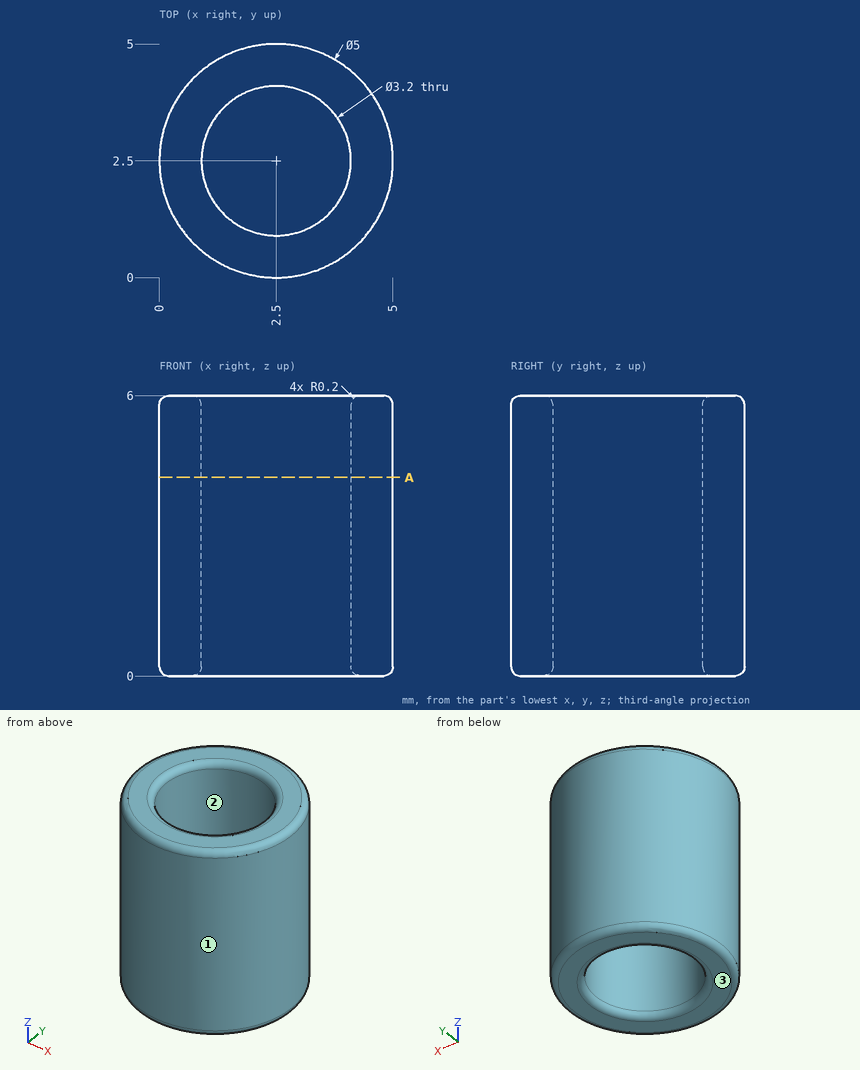
Study the drawing (mm; zero at the part's minimum x, y, z) and answer. Coordinates: 2 decimals unless noted, no trailing zeros. Write each loop counter-clockwise with the first axis right and the second up, starting at its lowest first coordinate (ties: lowest second). Pieces come first, ordered by that corner, then holes.
Q1. Given P1, Ø3, axis at x = 2.5, y = 2.5, coming from the +Z side; P2, Ø1.5, axis at x = 3.5, z = 4, coming from the +Y side, each flat-ended and moving along its own axis, determine where each tip first touches the part or whether it passes through.
Returned:
P1: passes through
P2: stops at y = 4.99
Q2. Find the intervals of material crossed by line 1 along Y through (x, z) = (2.45, 1.6); line 2 along Y through (x, z) = (3, 5.2); line 3 along X through (y, z) = (3.3, 5.4), in increasing order.
Returned:
line 1: y = 0 to 0.9, 4.1 to 5
line 2: y = 0.05 to 0.98, 4.02 to 4.95
line 3: x = 0.13 to 1.11, 3.89 to 4.87
Q3. The mould has two halves that part along Y. Classify the marked faces 1, 2 and 3: released by +Y, released by -Y, zero draft, split by the parting line, or undercut.
Returned:
face 1: split by the parting line
face 2: undercut
face 3: zero draft
Q4. Section A-A, the plane z = 4.25 is taken. Write down the section's boundary in (x, y), then the cut area to 3 significant figures.
Returned:
outline: circle Ø5 at (2.5, 2.5); hole circle Ø3.2 at (2.5, 2.5)
area: 11.6 mm2
